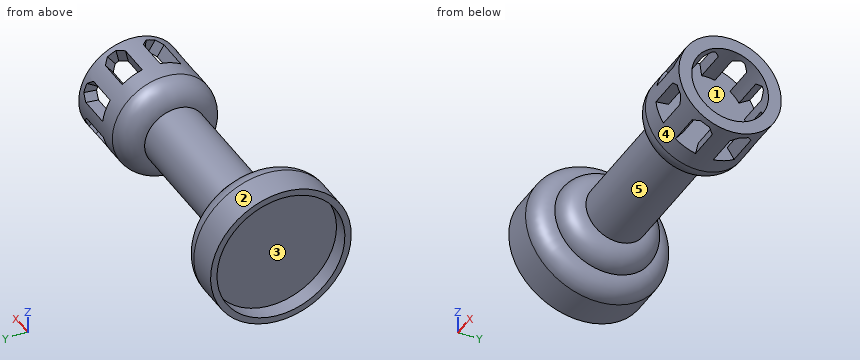
```python
from build123d import *

# Parameters (mm, degrees)
SKETCH_1_W               = 7
SKETCH_1_H               = 2
SKETCH_2_R               = 10
CUT_EXTRUDE_1_DEPTH      = 2.5
CUT_EXTRUDE_START        = 6
CUT_EXTRUDE_2_DEPTH      = 6
PATTERN_CIRCULAR_1_COUNT = 8
CHAMFER_4_SIZE           = 1
CHAMFER_5_SIZE           = 1
CHAMFER_6_SIZE           = 1


with BuildPart() as part:
    # Sketch 1 → Revolve 11 (revolve)
    with BuildSketch(Plane(origin=(0, 0, 0), x_dir=(1, 0, 0), z_dir=(0, 1, 0))):
        Polygon((5, 11), (0, 11), (0, 0), (5, 0), (5, 3), align=None)
        Polygon((8, 11), (5, 11), (5, 3), (8, 3), (8, 6.2), align=None)
        with BuildLine():
            Line((11.2, 6.2), (8, 6.2))
            Line((8, 6.2), (8, 3))
            ThreePointArc((8, 3), (10.2627417, 3.9372583), (11.2, 6.2))
        make_face()
        Polygon((35, 11), (8, 11), (8, 6.2), (11.2, 6.2), (31.465178427, 6.2), (35, 6.2), align=None)
        with BuildLine():
            Line((35, 3), (35, 6.2))
            Line((35, 6.2), (31.465178427, 6.2))
            ThreePointArc((31.465178427, 6.2), (32.615940251, 3.918829982), (35, 3))
        make_face()
        Polygon((38, 11), (35, 11), (35, 6.2), (35, 3), (38, 3), (38, 5), align=None)
        with Locations((41.5, 4)):
            Rectangle(SKETCH_1_W, SKETCH_1_H)
    revolve(axis=Axis((0, 0, -11), (1, 0, 0)))

    # Sketch 2 → Cut-Extrude 1 (cut)
    with BuildSketch(Plane.ZY):
        with Locations((-11, 0)):
            Circle(SKETCH_2_R)
    extrude(amount=-CUT_EXTRUDE_1_DEPTH, mode=Mode.SUBTRACT)

    # Sketch 6 → Cut-Extrude 2 (cut)
    with BuildSketch(Plane(origin=(38, 0, 0), x_dir=(0, 0, -1), z_dir=(1, 0, 0)).offset(CUT_EXTRUDE_START)):
        with BuildLine():
            Line((4.653173278, 4.870091432), (6.239879958, 3.652568574))
            ThreePointArc((6.239879958, 3.652568574), (5.562153278, 2.53570957), (5.142223957, 1.298637684))
            Line((5.142223957, 1.298637684), (3.189631943, 1.731516912))
            ThreePointArc((3.189631943, 1.731516912), (3.749537704, 3.380946094), (4.653173278, 4.870091432))
        make_face()
    cut_extrude_2 = extrude(amount=-CUT_EXTRUDE_2_DEPTH, mode=Mode.SUBTRACT)

    # Pattern Circular 1: Cut-Extrude 2 ×8 about axis
    pattern_circular_1_axis = Axis((0, 0, -11), (1, 0, 0))
    for i in range(1, PATTERN_CIRCULAR_1_COUNT):
        add(cut_extrude_2.rotate(pattern_circular_1_axis, i * 360 / PATTERN_CIRCULAR_1_COUNT), mode=Mode.SUBTRACT)

    # Sketch 1_12 → Revolve 12 (revolve)
    with BuildSketch(Plane(origin=(0, 0, 0), x_dir=(1, 0, 0), z_dir=(0, 1, 0))):
        with BuildLine():
            Line((5, 3), (5, 0))
            ThreePointArc((5, 0), (7.121320344, 0.878679656), (8, 3))
            Line((8, 3), (5, 3))
        make_face()
    revolve(axis=Axis((0, 0, -11), (1, 0, 0)))

    # Chamfer 4
    chamfer_4_edges = [part.edges().sort_by_distance(p)[0] for p in [
        (44, 3.761097258, -16.903740121),
        (44, 0.913683346, -17.94011403),
    ]]
    chamfer(chamfer_4_edges, length=CHAMFER_4_SIZE)

    # Chamfer 5
    chamfer_5_edges = [part.edges().sort_by_distance(p)[0] for p in [
        (44, 6.83407205, -12.515077298),
        (44, 5.553473382, -15.261330003),
    ]]
    chamfer(chamfer_5_edges, length=CHAMFER_5_SIZE)

    # Chamfer 6
    chamfer_6_edges = [part.edges().sort_by_distance(p)[0] for p in [
        (44, -1.515077298, -17.83407205),
        (44, -4.261330003, -16.553473382),
        (44, 5.903740121, -7.238902742),
        (44, 6.94011403, -10.086316654),
        (44, 1.515077298, -4.16592795),
        (44, 4.261330003, -5.446526618),
        (44, -3.761097258, -5.096259879),
        (44, -0.913683346, -4.05988597),
        (44, -6.83407205, -9.484922702),
        (44, -5.553473382, -6.738669997),
        (44, -5.903740121, -14.761097258),
        (44, -6.94011403, -11.913683346),
    ]]
    chamfer(chamfer_6_edges, length=CHAMFER_6_SIZE)


solid = part.part
```
Verification items for the finished model (mm, model axes). Face numbers are marked on the shaded views. A direction names the side the tool comes from. Give positions to 0.01 mm unless a question says otherwise; leave off trailing zeros. Order: outer loops, then holes, each group sorted by start corner. A loop starts at its lowest first (then second) coordinate and runs counter-clockwise, first axis right, second up. Notation, with made-up numbers: M 31.25,-33.75 L 40.25,-33.75 A37 cw 40.25,5.25 Z; hole C -2,5 d4. An arc over 180 degrees is marked long. Return JSON: item names as keys, results as strings. Group by question number.
1) Section check A-A on x = 40. Give the number of separate pieces and of enclosed holes in the cut face, and give its area (3 significant figures).
2) Section check D-D on x = 30. Record the cut outline in (y, z).
3) Section check C-C on z = -11. Record the cut outline in (x, y).
4) Scan lines: line 1 (Y direction, x = 1.5, z = -11); line 2 (Y direction, x = 41, z = -11); line 3 (Z direction, x = 42.75, y = 0). Record each from-to range of solid material in increasing order.
5) Section check B-B on y = 0. Record the cut outline in (x, z).
6) Mould release check, pull along X, two halves, no side actions. Record for the marked faces 1, 2 and 3: pulls with the +X half, pulls with the -X half, needs draft (parallel to the pull), parting line crosses it, or undercut.
7) Access from +Z, -Z, +X, -X, +Y, -Y to the whole of each face (thin tool, end or side, straight path). Record for the marked faces 4 and 5.
8) Go/stop test with flat-tipped pins: pin 1 Ø0.5 at (y, z) = (-3.5, -18) entering from -X; pin 2 Ø3 at (x, z) = (37, -7.5) entering from -Y; pin 3 Ø5 at (x, z) = (18.5, -14) entering from -Y. Record where each tip stops, or that it passes through.
Answer block:
{
 "1": {"separate pieces": "8", "enclosed holes": "0", "area": "39.1 mm^2"},
 "2": {"outline": "C 0,-11 d9.6"},
 "3": {"outline": "M 0,-11 L 5,-11 A3 ccw 8,-8 A3.2 ccw 11.2,-4.8 L 31.47,-4.8 A3.55 ccw 35,-8 L 45,-8 L 45,-6 L 38,-6 L 38,6 L 45,6 L 45,8 L 35,8 A3.55 ccw 31.47,4.8 L 11.2,4.8 A3.2 ccw 8,8 A3 ccw 5,11 L 0,11 L 0,10 L 2.5,10 L 2.5,-10 L 0,-10 Z"},
 "4": {"line 1": "y = -11 to -10, 10 to 11", "line 2": "y = -8 to -6, 6 to 8", "line 3": "z = -19 to -17, -5 to -3"},
 "5": {"outline": "M 0,-22 L 5,-22 A3 ccw 8,-19 A3.2 ccw 11.2,-15.8 L 31.47,-15.8 A3.55 ccw 35,-19 L 45,-19 L 45,-17 L 38,-17 L 38,-5 L 45,-5 L 45,-3 L 35,-3 A3.55 ccw 31.47,-6.2 L 11.2,-6.2 A3.2 ccw 8,-3 A3 ccw 5,0 L 0,0 L 0,-1 L 2.5,-1 L 2.5,-21 L 0,-21 Z"},
 "6": {"face 1": "undercut", "face 2": "needs draft", "face 3": "pulls with the -X half"},
 "7": {"face 4": "+X", "face 5": "none"},
 "8": {"pin 1": "stops at x = 2.5", "pin 2": "stops at y = -7.75", "pin 3": "stops at y = -4.77"}
}
